```python
from build123d import *

# Parameters (mm, degrees)
SKETCH1_R               = 25
BOSS_EXTRUDE1_DEPTH     = 10
CUT_EXTRUDE1_DEPTH      = 37.742346142
CUT_EXTRUDE1_DEPTH_BACK = 37.742346142
CUT_EXTRUDE2_DEPTH      = 3
SKETCH5_R               = 2
CUT_EXTRUDE4_DEPTH      = 13
FILLET1_R               = 1
CUT_EXTRUDE6_DEPTH      = 3
CUT_EXTRUDE6_DEPTH_BACK = 3
SKETCH6_W               = 10
SKETCH6_H               = 10
SKETCH7_W               = 10
SKETCH7_H               = 30
BOSS_EXTRUDE2_DEPTH     = 10
SKETCH8_W               = 10
SKETCH8_H               = 10
BOSS_EXTRUDE3_DEPTH     = 10
SKETCH9_W               = 10
SKETCH9_H               = 10
CUT_EXTRUDE7_DEPTH      = 10
SKETCH10_W              = 83.743898857
SKETCH10_H              = 28.854414255
SKETCH10_W_2            = 82.461079615
SKETCH10_H_2            = 26.234851391
CUT_EXTRUDE8_DEPTH      = 10
SKETCH11_W              = 10
SKETCH11_H              = 10.032703296
CUT_EXTRUDE9_DEPTH      = 10


with BuildPart() as part:
    # Sketch1 → Boss-Extrude1 (new body)
    with BuildSketch(Plane.XY):
        Circle(SKETCH1_R)
    extrude(amount=BOSS_EXTRUDE1_DEPTH)

    # Sketch2 → Cut-Extrude1 (cut, two sides: drawn at the far end of the back side and taken through both)
    with BuildSketch(Plane.XY.offset(10).offset(-CUT_EXTRUDE1_DEPTH_BACK)):
        Polygon((5, -5), (15, -5), (15, 5), (5, 5), (5, 15), (-5, 15), (-5, 5), (-15, 5), (-15, -5), (-5, -5), (-5, -15), (5, -15), align=None)
    extrude(amount=CUT_EXTRUDE1_DEPTH + CUT_EXTRUDE1_DEPTH_BACK, mode=Mode.SUBTRACT)

    # Sketch4 → Cut-Extrude2 (cut)
    with BuildSketch(Plane.ZY.offset(-15)):
        Polygon((4.759098318, -4.265594884), (8.57366269, -2.341424419), (8.814564373, 1.924170465), (5.240901682, 4.265594884), (1.42633731, 2.341424419), (1.185435627, -1.924170465), align=None)
    extrude(amount=-CUT_EXTRUDE2_DEPTH, mode=Mode.SUBTRACT)

    # Sketch5 → Cut-Extrude4 (cut)
    with BuildSketch(Plane.ZY.offset(-18)):
        with Locations((5, 0)):
            Circle(SKETCH5_R)
    extrude(amount=-CUT_EXTRUDE4_DEPTH, mode=Mode.SUBTRACT)

    # Fillet1
    fillet1_edges = [part.edges().sort_by_distance(p)[0] for p in [
        (-25, 0, 0),
        (-25, 0, 10),
    ]]
    fillet(fillet1_edges, radius=FILLET1_R)

    # Sketch6 → Cut-Extrude6 (cut, two sides: drawn at the far end of the back side and taken through both)
    with BuildSketch(Plane.YZ.offset(24.999151456).offset(-CUT_EXTRUDE6_DEPTH_BACK)):
        with Locations((0, 5)):
            Rectangle(SKETCH6_W, SKETCH6_H)
    extrude(amount=CUT_EXTRUDE6_DEPTH + CUT_EXTRUDE6_DEPTH_BACK, mode=Mode.SUBTRACT)

    # Sketch7 → Boss-Extrude2 (add)
    with BuildSketch(Plane(origin=(0, 0, 0), x_dir=(-1, 0, 0), z_dir=(0, 0, -1))):
        Rectangle(SKETCH7_W, SKETCH7_H)
    extrude(amount=-BOSS_EXTRUDE2_DEPTH)

    # Sketch8 → Boss-Extrude3 (add)
    with BuildSketch(Plane(origin=(0, 0, 0), x_dir=(-1, 0, 0), z_dir=(0, 0, -1))):
        with Locations((10, 0)):
            Rectangle(SKETCH8_W, SKETCH8_H)
    extrude(amount=-BOSS_EXTRUDE3_DEPTH)

    # Sketch9 → Cut-Extrude7 (cut)
    with BuildSketch(Plane(origin=(0, 0, 0), x_dir=(-1, 0, 0), z_dir=(0, 0, -1))):
        with Locations((15, 0)):
            Rectangle(SKETCH9_W, SKETCH9_H)
    extrude(amount=-CUT_EXTRUDE7_DEPTH, mode=Mode.SUBTRACT)

    # Sketch10 → Cut-Extrude8 (cut)
    with BuildSketch(Plane(origin=(0, 0, 0), x_dir=(-1, 0, 0), z_dir=(0, 0, -1))):
        with Locations((0.995128198, 24.427207128)):
            Rectangle(SKETCH10_W, SKETCH10_H)
        with Locations((-3.54772161, -23.117425695)):
            Rectangle(SKETCH10_W_2, SKETCH10_H_2)
    extrude(amount=-CUT_EXTRUDE8_DEPTH, mode=Mode.SUBTRACT)

    # Sketch11 → Cut-Extrude9 (cut)
    with BuildSketch(Plane(origin=(0, 0, 0), x_dir=(-1, 0, 0), z_dir=(0, 0, -1))):
        with Locations((-5, -0.016351648)):
            Rectangle(SKETCH11_W, SKETCH11_H)
    extrude(amount=-CUT_EXTRUDE9_DEPTH, mode=Mode.SUBTRACT)


solid = part.part
```
Geometry: final body of the model. Coordinates: model frame, mm. A direction names the side the tool comes from. Round coordinates to 2 decimals unless told otherwise and drop trailing zeros. Write each loop counter-clockwise with the first axis right and the second up, starting at its lowest first coordinate (ties: lowest second). Pieces come first, ordered by that corner, then holes.
Item 1: Set-up query: faces 5 (the face through (0, 10, 5)), 6 (the face through (16.48, -3.08, 2.95)), 7 (the face through (5, -5.033, 5)), 8 (the face through (23, -5, 5)). Return all of +Z, -Z, +X, -X, +Y, -Y with unobstructed straight access to the full face (end or side cutting, diameter ignored); none if empty.
Item 2: Section query D-D (y = 0). Return loops of the section in (x, z).
Item 3: Mould query, pull axis X, two halves, no side actions, for faces 1 (the face through (8, 5, 5)), 2 (the face through (-15, -5, 5)), 3 (the face through (23.824, -7.577, 4.944)), 4 (the face through (-5, 0, 10)). Classes: +X half, -X half, draft (parallel to the pull), parting line (faces both ways), or undercut.
Item 4: Pin query (flat end, axial travel): P1, Ø3, axis at y = 0, z = 3, coming from the +X side. Return the tip coordinate at first contact, or that it passes through.
Item 5: Section query A-A (x = 7). Return loops of the section in (y, z).
Item 6: Section query B-B (x = 15.5). Return loops of the section in (y, z).
Item 7: Material intervals for L1, parallel to Y at x = 7, z = 4.25; L2, parallel to X at y = -3.25, z = 7.5; L3, parallel to X at y = 1, z = 7.5, sorted ascending.
Completed:
1. face 5: +Z, -Z, +X, -X, +Y
1. face 6: none
1. face 7: +Z, -Z
1. face 8: +Z, -Z, +X
2. outline: (-25, 1) arc R1 ccw to (-24, 0) - (-20, 0) - (-20, 10) - (-24, 10) arc R1 ccw to (-25, 9) - close; (-10, 0) - (0, 0) - (0, 10) - (-10, 10) - close; (15, 0) - (22, 0) - (22, 3) - (18, 3) - (18, 1.29) - (15, 1.29) - close; (15, 8.71) - (18, 8.71) - (18, 7) - (22, 7) - (22, 10) - (15, 10) - close
3. face 1: undercut
3. face 2: undercut
3. face 3: +X half
3. face 4: draft
4. P1: stops at x = 22
5. outline: (-10, 0) - (-5.03, 0) - (-5.03, 10) - (-10, 10) - close; (5, 0) - (10, 0) - (10, 10) - (5, 10) - close
6. outline: (-10, 0) - (10, 0) - (10, 10) - (-10, 10) - close; hole (-4.27, 4.76) - (-1.92, 1.19) - (2.34, 1.43) - (4.27, 5.24) - (1.92, 8.81) - (-2.34, 8.57) - close
7. L1: y = -10 to -5.03, 5 to 10
7. L2: x = -24.79 to -20, -10 to 0, 15 to 22
7. L3: x = -24.98 to -20, -10 to 0, 18 to 22
